Verification items for the finished model (mm, model axes). Coordinates: 2 decimals unless noted, no trailing zeros. Order: outer loops, then holes, each group sorted by start corner. A loop starts at its lowest first (then second) coordinate and runs counter-clockwise, first axis right, second up.
Q1. Cross-section at A-A, the plane y = 1.25. Record the boundary of the cut face in (x, z) (3 decimals), and give its area (3 significant figures).
Q2. Thickness scan on line 1 (X direction, y = 2, z = -81) (3 decimals); line 2 (Z direction, x = 1, y = -0.25). Record the ranges inside material, lowest first.
Q3. Depth check by flat-ended pin: P1, Ø3, axis at x = 1.5, y = 1, coming from the -Z side. Enter the tip coordinate at first touch or a pass-through.
from build123d import *

# Parameters (mm, degrees)
F0_W     = 50
F0_H     = 197.460108
F1_DEPTH = 3.175
F4_W     = 6.35
F4_H     = 25
F5_DEPTH = 6.351


with BuildPart() as f1:
    # F0 (on Front) → F1 (new body, symmetric)
    with BuildSketch(Plane.XZ):
        Rectangle(F0_W, F0_H)
    extrude(amount=F1_DEPTH, both=True)

    # F2 (on face) → F3 (revolve, cut)
    with BuildSketch(Plane.XZ.offset(3.175)):
        with BuildLine():
            ThreePointArc((0, 71.230054), (2.5, 73.730054), (0, 76.230054))
            Line((0, 76.230054), (0, 71.230054))
        make_face()
    revolve(axis=Axis((0, -3.175, 73.730054), (0, 0, -1)), mode=Mode.SUBTRACT)

    # F4 (on face) → F5 (cut, through all)
    with BuildSketch(Plane.XZ.offset(3.175)):
        with Locations((0, -86.230054)):
            Rectangle(F4_W, F4_H)
    extrude(amount=-F5_DEPTH, mode=Mode.SUBTRACT)


solid = f1.part
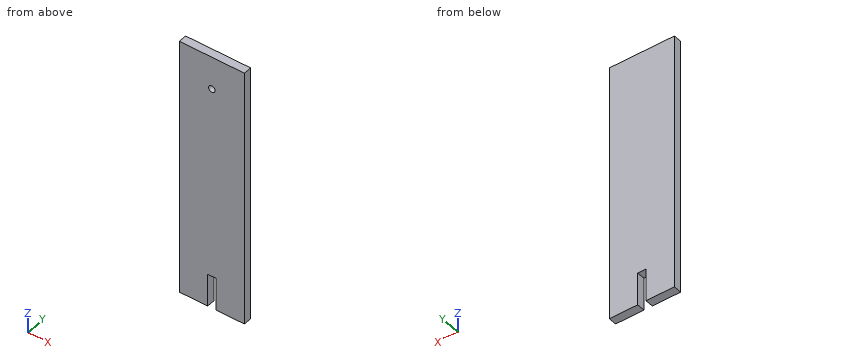
Check values:
1. outline: (-25, -98.73) - (-3.175, -98.73) - (-3.175, -73.73) - (3.175, -73.73) - (3.175, -98.73) - (25, -98.73) - (25, 98.73) - (-25, 98.73) - close
1. area: 9,710 mm2
2. line 1: x = -25 to -3.175, 3.175 to 25
2. line 2: z = -73.73 to 98.73
3. P1: stops at z = -73.73
